from build123d import *

# Parameters (mm, degrees)
SM_BASE_FLANGE_1_DEPTH = 55
OTHER_START            = -1
OTHER_1_DEPTH          = 2
OTHER_START_2          = 1
OTHER_1_2_DEPTH        = 79
OTHER_START_3          = -0.24719
OTHER_1_3_DEPTH        = 81.24719
OTHER_START_4          = -51.5
OTHER_1_4_DEPTH        = 103
OTHER_1_5_DEPTH        = 103
SM_EDGE_FLANGE_1_DEPTH = 98
SKETCH_19_W            = 10
SKETCH_19_H            = 10
CUT_EXTRUDE_1_DEPTH    = 1.5
SM_EDGE_FLANGE_2_DEPTH = 8
SKETCH_24_R            = 1.5
CUT_EXTRUDE_2_DEPTH    = 0.5
SKETCH_27_W            = 3
SKETCH_27_H            = 10
CUT_EXTRUDE_3_DEPTH    = 0.5


with BuildPart() as part:
    # 基体-法兰1: sheet metal written as solids
    # Sketch 1 → 基体-法兰1 (new, symmetric)
    with BuildSketch(Plane.XY):
        with BuildLine():
            Line((-52.5, 80), (-52.5, 1))
            ThreePointArc((-52.5, 1), (-52.207106781, 0.292893219), (-51.5, 0))
            Line((-51.5, 0), (51.5, 0))
            ThreePointArc((51.5, 0), (52.207106781, 0.292893219), (52.5, 1))
            Line((52.5, 1), (52.5, 80))
            Line((52.5, 80), (53, 80))
            Line((53, 80), (53, 1))
            ThreePointArc((53, 1), (52.560660172, -0.060660172), (51.5, -0.5))
            Line((51.5, -0.5), (-51.5, -0.5))
            ThreePointArc((-51.5, -0.5), (-52.560660172, -0.060660172), (-53, 1))
            Line((-53, 1), (-53, 80))
            Line((-53, 80), (-52.5, 80))
        make_face()
    extrude(amount=SM_BASE_FLANGE_1_DEPTH, both=True)

    # Other 1: read off the stored shape, not the designer's step
    # Other 1 outline → Other 1 (cut)
    with BuildSketch(Plane(origin=(0, 0, 0), x_dir=(1, 0, 0), z_dir=(0, 1, 0)).offset(OTHER_START)):
        with BuildLine():
            Line((51.5, -54.45), (51.5, -55))
            Line((51.5, -55), (52.45, -55))
            ThreePointArc((52.45, -55), (52.83890873, -54.83890873), (53, -54.45))
            Line((53, -54.45), (51.5, -54.45))
        make_face()
        with BuildLine():
            Line((-52.45, -55), (-51.5, -55))
            Line((-51.5, -55), (-51.5, -54.45))
            Line((-51.5, -54.45), (-53, -54.45))
            ThreePointArc((-53, -54.45), (-52.83890873, -54.83890873), (-52.45, -55))
        make_face()
    extrude(amount=OTHER_1_DEPTH, mode=Mode.SUBTRACT)

    # Other 1 2 outline → Other 1 2 (add)
    with BuildSketch(Plane(origin=(0, 0, 0), x_dir=(1, 0, 0), z_dir=(0, 1, 0)).offset(OTHER_START_2)):
        with BuildLine():
            Line((51.9, -45), (51.9, -54.45))
            ThreePointArc((51.9, -54.45), (52.45, -55), (53, -54.45))
            Line((53, -54.45), (52.5, -54.45))
            ThreePointArc((52.5, -54.45), (52.45, -54.5), (52.4, -54.45))
            Line((52.4, -54.45), (52.4, -45))
            Line((52.4, -45), (51.9, -45))
        make_face()
        with BuildLine():
            ThreePointArc((-53, -54.45), (-52.45, -55), (-51.9, -54.45))
            Line((-51.9, -54.45), (-51.9, -45))
            Line((-51.9, -45), (-52.4, -45))
            Line((-52.4, -45), (-52.4, -54.45))
            ThreePointArc((-52.4, -54.45), (-52.45, -54.5), (-52.5, -54.45))
            Line((-52.5, -54.45), (-53, -54.45))
        make_face()
    extrude(amount=OTHER_1_2_DEPTH)

    # Other 1 3 outline → Other 1 3 (cut)
    with BuildSketch(Plane(origin=(0, 0, 0), x_dir=(1, 0, 0), z_dir=(0, 1, 0)).offset(OTHER_START_3)):
        with BuildLine():
            ThreePointArc((-52.45, -55), (-52.83890873, -54.83890873), (-53, -54.45))
            Line((-53, -54.45), (-53, -55))
            Line((-53, -55), (-52.45, -55))
        make_face()
        with BuildLine():
            Line((52.45, -55), (53, -55))
            Line((53, -55), (53, -54.45))
            ThreePointArc((53, -54.45), (52.83890873, -54.83890873), (52.45, -55))
        make_face()
    extrude(amount=OTHER_1_3_DEPTH, mode=Mode.SUBTRACT)

    # Other 1 4 outline → Other 1 4 (cut)
    with BuildSketch(Plane.YZ.offset(OTHER_START_4)):
        with BuildLine():
            ThreePointArc((-0.5, 54.45), (-0.35620192, 54.820809924), (0, 54.997722558))
            Line((0, 54.997722558), (0, 55))
            Line((0, 55), (-0.5, 55))
            Line((-0.5, 55), (-0.5, 54.45))
        make_face()
    extrude(amount=OTHER_1_4_DEPTH, mode=Mode.SUBTRACT)

    # Other 1 5 outline → Other 1 5 (add)
    with BuildSketch(Plane.YZ.offset(OTHER_START_4)):
        with BuildLine():
            Line((0.1, 45), (0.6, 45))
            Line((0.6, 45), (0.6, 54.45))
            ThreePointArc((0.6, 54.45), (0.420809924, 54.85620192), (0, 54.997722558))
            Line((0, 54.997722558), (0, 54.45))
            ThreePointArc((0, 54.45), (0.05, 54.5), (0.1, 54.45))
            Line((0.1, 54.45), (0.1, 45))
        make_face()
    extrude(amount=OTHER_1_5_DEPTH)

    # 边线-法兰1: sheet metal written as solids
    # 边线-法兰1 section (on a plane across the edge) → 边线-法兰1 (add)
    with BuildSketch(Plane(origin=(-52.5, 81, -55), x_dir=(0, -1, 0), z_dir=(0, 0, 1))):
        with BuildLine():
            Line((-0.5, 1), (-0.5, 9.5))
            Line((-0.5, 9.5), (0, 9.5))
            Line((0, 9.5), (0, 1))
            ThreePointArc((0, 1), (0.292893219, 0.292893219), (1, 0))
            Line((1, 0), (1, -0.5))
            ThreePointArc((1, -0.5), (-0.060660172, -0.060660172), (-0.5, 1))
        make_face()
    sm_edge_flange_1 = extrude(amount=SM_EDGE_FLANGE_1_DEPTH)

    # 镜向1: 边线-法兰1 across plane
    add(sm_edge_flange_1.mirror(Plane(origin=(0, 0, 0), x_dir=(0, 0, 1), z_dir=(1, 0, 0))))

    # 草图19 → 切除-拉伸1 (cut)
    with BuildSketch(Plane(origin=(0, 81.5, 0), x_dir=(1, 0, 0), z_dir=(0, 1, 0))):
        with Locations((50, 10)):
            Rectangle(SKETCH_19_W, SKETCH_19_H)
    extrude(amount=-CUT_EXTRUDE_1_DEPTH, mode=Mode.SUBTRACT)

    # 边线-法兰2: sheet metal written as solids
    # 边线-法兰2 section (on a plane across the edge) → 边线-法兰2 (add)
    with BuildSketch(Plane(origin=(53, 81, -14), x_dir=(0, -1, 0), z_dir=(0, 0, 1))):
        with BuildLine():
            Line((-0.5, 1), (-0.5, 5.5))
            Line((-0.5, 5.5), (0, 5.5))
            Line((0, 5.5), (0, 1))
            ThreePointArc((0, 1), (0.292893219, 0.292893219), (1, 0))
            Line((1, 0), (1, -0.5))
            ThreePointArc((1, -0.5), (-0.060660172, -0.060660172), (-0.5, 1))
        make_face()
    extrude(amount=SM_EDGE_FLANGE_2_DEPTH)

    # 草图24 → 切除-拉伸2 (cut)
    with BuildSketch(Plane(origin=(0, 81.5, 0), x_dir=(1, 0, 0), z_dir=(0, 1, 0))):
        with Locations(Location((56, 10, 0), (0, 0, 180))):
            Circle(SKETCH_24_R)
    extrude(amount=-CUT_EXTRUDE_2_DEPTH, mode=Mode.SUBTRACT)

    # 草图27 → 切除-拉伸3 (cut)
    with BuildSketch(Plane(origin=(0, 81.5, 0), x_dir=(1, 0, 0), z_dir=(0, 1, 0))):
        with Locations((47.5, 35)):
            Rectangle(SKETCH_27_W, SKETCH_27_H)
        with Locations((47.5, -15)):
            Rectangle(SKETCH_27_W, SKETCH_27_H)
        with Locations((-47.5, 35)):
            Rectangle(SKETCH_27_W, SKETCH_27_H)
        with Locations((-47.5, -15)):
            Rectangle(SKETCH_27_W, SKETCH_27_H)
    extrude(amount=-CUT_EXTRUDE_3_DEPTH, mode=Mode.SUBTRACT)


solid = part.part
Source: CAD feature listing. Evaluate the final solid. Frame: model axes, mm. A direction names the side the tool comes from. Give positions to 0.01 mm unless a question says otherwise; leave off trailing zeros. Write each loop counter-clockwise with the first axis right and the second up, starting at its lowest first coordinate (ties: lowest second). Pieces come first, ordered by that corner, then holes. Notation, with made-up numbers: M 26.25,88 L 55.25,88 A21 ccw 55.25,119 Z; hole C -7,9.25 d8. An arc over 180 degrees is marked long. Answer as a JSON object with one key per item and string values.
Q1. Contact query for flat-ended pins moving along their axis: P1, Ø5, axis at x = 57.5, z = -12, coming from the -Y side; P2, Ø2, axis at y = 48, z = -10, coming from the +X side; P3, Ø0.9, axis at x = -52.5, z = 49.5, coming from the +Y side. Output: stop coordinate, or through.
Geometry check:
{"P1": "stops at y = 81", "P2": "stops at x = 53", "P3": "stops at y = 80"}
Q2. Cut plane B-B, the plane x = 56. Return the cut outline in (y, z), then the cut area to 3 significant figures.
Geometry check:
{"outline": "M 81,-14 L 81.5,-14 L 81.5,-11.5 L 81,-11.5 Z; M 81,-8.5 L 81.5,-8.5 L 81.5,-6 L 81,-6 Z", "area": "2.50 mm^2"}
Q3. Cut plane C-C, the plane z = 32. Return the cut outline in (x, y).
Geometry check:
{"outline": "M -53,1 A1.5 ccw -51.5,-0.5 L 51.5,-0.5 A1.5 ccw 53,1 L 53,80 A1.5 ccw 51.5,81.5 L 43,81.5 L 43,81 L 51.5,81 A1 cw 52.5,80 L 52.5,1 A1 cw 51.5,0 L -51.5,0 A1 cw -52.5,1 L -52.5,80 A1 cw -51.5,81 L -43,81 L -43,81.5 L -51.5,81.5 A1.5 ccw -53,80 Z"}
Q4. Access query for faces 5 (the face through (58, 81, -10)), 6 (the face through (-47, 81, -7)), 7 (the face through (58, 81.5, -10)), 8 (the face through (-1, 0.6, 50)). Directions: +Z, -Z, +X, -X, +Y, -Y. A direction counts if a zero-diameter tool reaches every point of the face in a straight line with its end or side. Return the directions, or none.
Geometry check:
{"face 5": "+Z, -Z, +X, -Y", "face 6": "+Z, -Z", "face 7": "+Z, -Z, +X, -X, +Y", "face 8": "+Z, -Z, +Y"}
Q5. Cut plane A-A, the plane y = 49. Return the cut outline in (x, z), then the cut area to 3 significant figures.
Geometry check:
{"outline": "M -53,-55 L -52.5,-55 L -52.5,54.45 A0.05 cw -52.4,54.45 L -52.4,45 L -51.9,45 L -51.9,54.45 A0.55 ccw -53,54.45 Z; M 51.9,45 L 52.4,45 L 52.4,54.45 A0.05 cw 52.5,54.45 L 52.5,-55 L 53,-55 L 53,54.45 A0.55 ccw 51.9,54.45 Z", "area": "120 mm^2"}
Q6. Ray query, line 1 along Z through (x, y) = (56, 81.3); line 2 along X through (y, z) = (7, -12); line 3 along Y through (x, z) = (-24, -30.5). Return the intervals inside material, ascending.
Geometry check:
{"line 1": "z = -14 to -11.5, -8.5 to -6", "line 2": "x = -53 to -52.5, 52.5 to 53", "line 3": "y = -0.5 to 0"}
Q7. Mould query, pull axis X, two halves, no side actions, for faces 1 (the face through (44, 81.5, -7)), 2 (the face through (53, 41, 0)), 3 (the face through (-53, 40, 0)), 4 (the face through (51.9, 40, 50)). Classes: +X half, -X half, draft (parallel to the pull), parting line (faces both ways), or undercut.
Geometry check:
{"face 1": "draft", "face 2": "+X half", "face 3": "-X half", "face 4": "undercut"}
Q8. Cut plane D-D, the plane x = -12. Return the cut outline in (y, z).
Geometry check:
{"outline": "M -0.5,-55 L 0,-55 L 0,54.45 A0.05 cw 0.1,54.45 L 0.1,45 L 0.6,45 L 0.6,54.45 A0.55 ccw -0.5,54.45 Z"}
